Verification items for the finished model (mm, model axes). Face numbers are marked on the shaded views. Round coordinates to 2 decimals unless told otherwise and drop trailing zeros. Write each loop counter-clockwise with the first axis right and the second up, starting at its lowest first coordinate (ties: lowest second). Pieces come first, ordered by that corner, then holes. Notation, with made-up numbers: M 1,-20.5 L 51,-20.5 A30 cw 51,5.5 Z; hole C 20,-29 d6. An arc over 180 degrees is marked long. One line per question, with ' | ' between items.
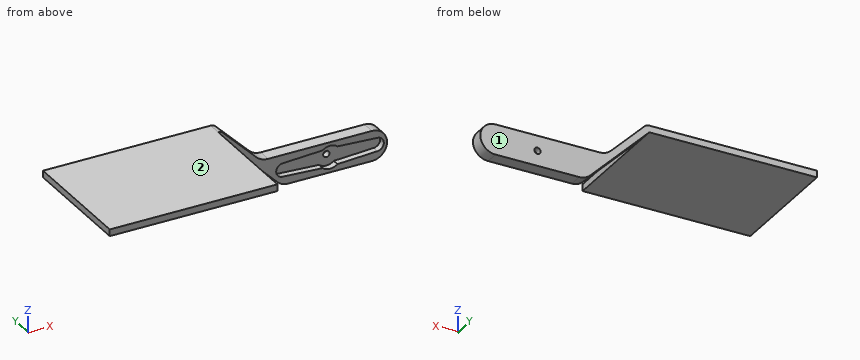
from build123d import *

# Parameters (mm, degrees)
RESSALTO_EXTRUS_O1_DEPTH = 4
ESBO_O2_W                = 50
ESBO_O2_H                = 2
RESSALTO_EXTRUS_O2_DEPTH = 32
ESBO_O3_R                = 0.94
CORTE_EXTRUS_O1_DEPTH    = 37
CORTE_EXTRUS_O2_DEPTH    = 2
FILETE1_R                = 2


with BuildPart() as part:
    # Esboço1 → Ressalto-extrusão1 (new body)
    with BuildSketch(Plane(origin=(0, 0, 0), x_dir=(1, 0, 0), z_dir=(0, 1, 0))):
        with BuildLine():
            Line((12.5, 4.5), (-12.5, 4.5))
            ThreePointArc((-12.5, 4.5), (-14.222075446, 4.157457896), (-15.681980515, 3.181980515))
            Line((-15.681980515, 3.181980515), (-33.359650045, -14.495689014))
            Line((-33.359650045, -14.495689014), (-83.359650045, -14.495689014))
            Line((-83.359650045, -14.495689014), (-83.359650045, -16.495689014))
            Line((-83.359650045, -16.495689014), (-32.53122292, -16.495689014))
            Line((-32.53122292, -16.495689014), (-22, -5.964466094))
            ThreePointArc((-22, -5.964466094), (-20.377883256, -4.880602337), (-18.464466094, -4.5))
            Line((-18.464466094, -4.5), (12.5, -4.5))
            ThreePointArc((12.5, -4.5), (17, 0), (12.5, 4.5))
        make_face()
    extrude(amount=-RESSALTO_EXTRUS_O1_DEPTH)

    # Esboço2 → Ressalto-extrusão2 (add)
    with BuildSketch(Plane.XZ.offset(4)):
        with Locations((-58.359650045, 15.495689014)):
            Rectangle(ESBO_O2_W, ESBO_O2_H)
    extrude(amount=RESSALTO_EXTRUS_O2_DEPTH)

    # Esboço3 → Corte-extrusão1 (cut, through all)
    with BuildSketch(Plane(origin=(0, 0, 0), x_dir=(1, 0, 0), z_dir=(0, 1, 0))):
        Circle(ESBO_O3_R)
    extrude(amount=-CORTE_EXTRUS_O1_DEPTH, mode=Mode.SUBTRACT)

    # Esboço6 → Corte-extrusão2 (cut)
    with BuildSketch(Plane(origin=(0, -4, 0), x_dir=(1, 0, 0), z_dir=(0, 1, 0))):
        with BuildLine():
            Line((-14.05, 2), (-2.209072203, 2.65))
            ThreePointArc((-2.209072203, 2.65), (0, 3.45), (2.209072203, 2.65))
            Line((2.209072203, 2.65), (14.05, 2))
            ThreePointArc((14.05, 2), (16.05, 0), (14.05, -2))
            Line((14.05, -2), (2.209072203, -2.65))
            ThreePointArc((2.209072203, -2.65), (0, -3.45), (-2.209072203, -2.65))
            Line((-2.209072203, -2.65), (-14.05, -2))
            ThreePointArc((-14.05, -2), (-16.05, 0), (-14.05, 2))
        make_face()
    extrude(amount=CORTE_EXTRUS_O2_DEPTH, mode=Mode.SUBTRACT)

    # Filete1
    filete1_edges = [part.edges().sort_by_distance(p)[0] for p in [
        (-32.53122292, -2, 16.495689014),
    ]]
    fillet(filete1_edges, radius=FILETE1_R)


solid = part.part
1. Section check C-C, the plane y = -25. Record the cut outline in (x, z), then the cut area to 3 significant figures.
Results:
outline: M -83.36,14.5 L -33.36,14.5 L -33.36,16.5 L -83.36,16.5 Z | area: 100 mm2
2. Go/stop test with flat-tipped pins: P1, Ø3, axis at x = 0, y = -2.5, coming from the +Z side; P2, Ø12, axis at y = -28.5, z = 2.5, coming from the -X side; P3, Ø8, axis at x = -55, y = -15.5, coming from the -Z side; P4, Ø1, axis at y = -24.5, z = 15.5, coming from the +X side. Record where each tip stops, or that it passes through.
Results:
P1: stops at z = 4.5 | P2: passes through | P3: stops at z = 14.5 | P4: stops at x = -33.36
3. Section check A-A, the plane x = 0. Record the cut outline in (y, z), then the cut area to 3 significant figures.
Results:
outline: M -4,-4.5 L 0,-4.5 L 0,-0.94 L -2,-0.94 L -2,-3.45 L -4,-3.45 Z; M -4,3.45 L -2,3.45 L -2,0.94 L 0,0.94 L 0,4.5 L -4,4.5 Z | area: 18.4 mm2
4. Section check D-D, the plane x = -73. Record the cut outline in (y, z).
Results:
outline: M -36,14.5 L 0,14.5 L 0,16.5 L -36,16.5 Z
5. Thickness scan on line 1 (Z direction, x = 0, y = -1.5); line 2 (Z direction, x = -65, y = -34); line 3 (X direction, y = -0.7, z = 0). Record the ranges inside material, lowest first.
Results:
line 1: z = -4.5 to -0.94, 0.94 to 4.5 | line 2: z = 14.5 to 16.5 | line 3: x = -18.86 to -0.94, 0.94 to 17
6. Mould release check, pull along Y, two halves, no side actions. Record for the marked faces 1 and 2: pulls with the +Y half, pulls with the -Y half, needs draft (parallel to the pull), parting line crosses it, or undercut.
Results:
face 1: pulls with the +Y half | face 2: needs draft
7. Section check B-B, the plane z = 0. Record the cut outline in (x, y), then the cut area to 3 significant figures.
Results:
outline: M -18.86,-4 L -16.05,-4 L -16.05,-2 L -0.94,-2 L -0.94,0 L -18.86,0 Z; M 0.94,-2 L 16.05,-2 L 16.05,-4 L 17,-4 L 17,0 L 0.94,0 Z | area: 75.5 mm2
